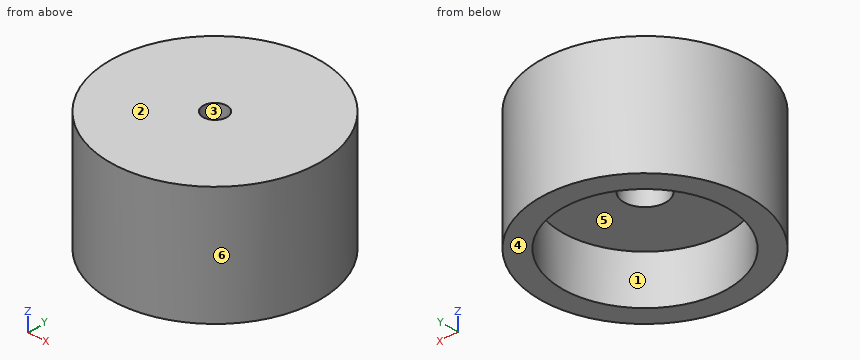
```python
from build123d import *

# Parameters (mm, degrees)
CYLINDER091_R     = 3
CYLINDER091_DEPTH = 10
CYLINDER090_R     = 1.7
CYLINDER090_DEPTH = 30
CYLINDER092_R     = 11.85
CYLINDER092_DEPTH = 100
CYLINDER014_R     = 15
CYLINDER014_DEPTH = 17


with BuildPart() as cylinder369:
    # Cylinder091 → Cylinder091 (new body)
    with BuildSketch(Plane.XY.offset(124)):
        Circle(CYLINDER091_R)
    extrude(amount=CYLINDER091_DEPTH)


with BuildPart() as cylinder368:
    # Cylinder090 → Cylinder090 (new body)
    with BuildSketch(Plane.XY.offset(128)):
        Circle(CYLINDER090_R)
    extrude(amount=CYLINDER090_DEPTH)


with BuildPart() as cylinder370:
    # Cylinder092 → Cylinder092 (new body)
    with BuildSketch(Plane.XY.offset(31)):
        Circle(CYLINDER092_R)
    extrude(amount=CYLINDER092_DEPTH)


with BuildPart() as winder_end_free:
    # Cylinder014 → Cylinder014 (new body)
    with BuildSketch(Plane.XY.offset(124)):
        Circle(CYLINDER014_R)
    extrude(amount=CYLINDER014_DEPTH)

    # Cut050: cut Cylinder370
    add(cylinder370.part, mode=Mode.SUBTRACT)

    # Cut051: cut Cylinder368
    add(cylinder368.part, mode=Mode.SUBTRACT)

    # Cut052: cut Cylinder369
    add(cylinder369.part, mode=Mode.SUBTRACT)


solid = winder_end_free.part
```
The listing builds one solid part. Answer for the finished solid, in the listing's coordinates (mm). Face numbers are marked on the shaded views. A direction names the side the tool comes from. Round coordinates to 2 decimals unless told otherwise and drop trailing zeros. Loops run counter-clockwise (first coordinate to the right, second up) from the corner with the lowest first, then second, coordinate; pieces in that order, holes last.
1) For a pull along X with two mould halves and no side action, classify the marked faces 3, 4, 5 and 6 as released by +X, released by -X, zero draft, split by the parting line, or undercut.
Outcome:
face 3: undercut
face 4: zero draft
face 5: undercut
face 6: split by the parting line
2) Consider line 1 (Y direction, x = 0, z = 132.45); line 2 (Y direction, x = 0, z = 137.5); line 3 (Z direction, x = 4.25, y = 8.75). Determine where each line is inside the solid, lowest interval first.
Outcome:
line 1: y = -15 to -3, 3 to 15
line 2: y = -15 to -1.7, 1.7 to 15
line 3: z = 131 to 141
3) A cutting plane is placed at A-A on x = 0. Determine the outline of the cut face in (y, z), plus the area to 3 significant figures.
Outcome:
outline: (-15, 124) - (-11.85, 124) - (-11.85, 131) - (-3, 131) - (-3, 134) - (-1.7, 134) - (-1.7, 141) - (-15, 141) - close; (1.7, 134) - (3, 134) - (3, 131) - (11.85, 131) - (11.85, 124) - (15, 124) - (15, 141) - (1.7, 141) - close
area: 302 mm2
4) A cutting plane is placed at D-D on x = -10. Determine the outline of the cut face in (y, z), plus the area to 3 significant figures.
Outcome:
outline: (-11.18, 124) - (-6.36, 124) - (-6.36, 131) - (6.36, 131) - (6.36, 124) - (11.18, 124) - (11.18, 141) - (-11.18, 141) - close
area: 291 mm2
5) For the marked faces 1 and 2, determine the directions among +Z, -Z, +X, -X, +Y, -Y from which every point of the face is accessible in a straight line to the end or side of a thin tool.
Outcome:
face 1: -Z
face 2: +Z, +X, -X, +Y, -Y
6) A cutting plane is placed at C-C on z = 132.5. Determine the outline of the cut face in (x, y), plus the area to 3 significant figures.
Outcome:
outline: circle Ø30 at (0, 0); hole circle Ø6 at (0, 0)
area: 679 mm2
7) Given P1, Ø7, axis at x = -3.5, y = -3, coming from the -Z side; P2, Ø5.5, axis at x = 0, y = 0, coming from the -Z side; P3, Ø6, axis at y = -6.5, z = 128.5, coming from the -X side, each flat-ended and moving along its own axis, determine where each tip first touches the part or whether it passes through.
Outcome:
P1: stops at z = 131
P2: stops at z = 134
P3: stops at x = -14.59
